Input: part model. Units: mm. Frame: model coordinates. Coordinates: 2 decimals unless noted, no trailing zeros. Write each loop counter-clockwise with the first axis right and the second up, starting at its lowest first coordinate (ties: lowest second). Pieces come first, ordered by that corner, then holes.
1) Section query B-B (y = 10). Output: boundary loops of the cut face in (x, z), then the cut area to 3 significant figures.
2) Line query: L1, parallel to Y at x = 65.75, z = 4.25; L2, parallel to Y at x = 127, z = 4.25; L3, parallel to Y at x = 102.5, z = 1. Output: solid intervals per line, ascending.
3) Pin query (flat end, axial travel): pin 1 Ø2.5 at (x, y) = (-5.06, 36) entering from -Z; pin 2 Ø0.6 at (x, z) = (150.5, 1.5) entering from -Y; pin 3 Ø2 at (x, y) = (45, 14.5) entering from +Z; pin 4 Ø1 at (y, z) = (-24.5, 1.5) entering from -X. Return the tip coordinate at first contact, or that it passes through.
4) Section query C-C (z = 4.25). State how many separate pieces and enclosed holes the cut face has, then the cut area to 3 significant figures.
5) Section query A-A (x = 123). Output: boundary loops of the cut face in (y, z), then the cut area to 3 significant figures.
from build123d import *

# Parameters (mm, degrees)
SKETCH_R     = 17.5
PAD_DEPTH    = 2
SKETCH002_W  = 10
SKETCH002_H  = 2
PAD003_DEPTH = 10
SKETCH003_W  = 10
SKETCH003_H  = 2
PAD004_DEPTH = 10
SKETCH006_W  = 10
SKETCH006_H  = 2
PAD007_DEPTH = 10
SKETCH001_R  = 2.5
PAD006_DEPTH = 5
SKETCH005_R  = 1.5
POCKET_DEPTH = 7.001


with BuildPart() as part:
    # Sketch → Pad (new body)
    with BuildSketch(Plane.XY):
        Polygon((0, 0), (0, 20.5), (0, 41), (20.5, 41), (41, 41), (61.5, 41), (82, 41), (102.5, 41), (82, 41), (102.5, 41), (123, 41), (143.5, 41), (164, 41), (164, 20.5), (164, 0), (143.5, 0), (143.5, -20.5), (143.5, -41), (123, -41), (102.5, -41), (82, -41), (61.5, -41), (41, -41), (20.5, -41), (20.5, -20.5), (20.5, 0), align=None)
        with Locations((20.5, 20.5)):
            Circle(SKETCH_R, mode=Mode.SUBTRACT)
        with Locations((61.5, 20.5)):
            Circle(SKETCH_R, mode=Mode.SUBTRACT)
        with Locations((102.5, 20.5)):
            Circle(SKETCH_R, mode=Mode.SUBTRACT)
        with Locations((143.5, 20.5)):
            Circle(SKETCH_R, mode=Mode.SUBTRACT)
        with Locations((41, -20.5)):
            Circle(SKETCH_R, mode=Mode.SUBTRACT)
        with Locations((82, -20.5)):
            Circle(SKETCH_R, mode=Mode.SUBTRACT)
        with Locations((123, -20.5)):
            Circle(SKETCH_R, mode=Mode.SUBTRACT)
    extrude(amount=PAD_DEPTH)

    # Sketch002 → Pad003 (join)
    with BuildSketch(Plane(origin=(0, 0, 0), x_dir=(0, -1, 0), z_dir=(-1, 0, 0))):
        with Locations((-36, 1)):
            Rectangle(SKETCH002_W, SKETCH002_H)
    extrude(amount=PAD003_DEPTH)

    # Sketch003 (on Face14 of Pad003) → Pad004 (join)
    with BuildSketch(Plane.XZ.offset(41)):
        with Locations((138.5, 1)):
            Rectangle(SKETCH003_W, SKETCH003_H)
    extrude(amount=PAD004_DEPTH)

    # Sketch006 (on Face8 of Pad004) → Pad007 (join)
    with BuildSketch(Plane(origin=(0, 41, 0), x_dir=(-1, 0, 0), z_dir=(0, 1, 0))):
        with Locations((-159, 1)):
            Rectangle(SKETCH006_W, SKETCH006_H)
    extrude(amount=PAD007_DEPTH)

    # Sketch001 (on Face35 of Pad) → Pad006 (join)
    with BuildSketch(Plane.XY.offset(2)):
        with Locations((4.25, 36.75)):
            Circle(SKETCH001_R)
        with Locations((36.75, 36.75)):
            Circle(SKETCH001_R)
        with Locations((4.25, 4.25)):
            Circle(SKETCH001_R)
        with Locations((36.75, 4.25)):
            Circle(SKETCH001_R)
        with Locations((45.25, 36.75)):
            Circle(SKETCH001_R)
        with Locations((77.75, 36.75)):
            Circle(SKETCH001_R)
        with Locations((45.25, 4.25)):
            Circle(SKETCH001_R)
        with Locations((77.75, 4.25)):
            Circle(SKETCH001_R)
        with Locations((86.25, 36.75)):
            Circle(SKETCH001_R)
        with Locations((118.75, 36.75)):
            Circle(SKETCH001_R)
        with Locations((86.25, 4.25)):
            Circle(SKETCH001_R)
        with Locations((118.75, 4.25)):
            Circle(SKETCH001_R)
        with Locations((127.25, 36.75)):
            Circle(SKETCH001_R)
        with Locations((159.75, 36.75)):
            Circle(SKETCH001_R)
        with Locations((127.25, 4.25)):
            Circle(SKETCH001_R)
        with Locations((159.75, 4.25)):
            Circle(SKETCH001_R)
        with Locations((24.75, -4.25)):
            Circle(SKETCH001_R)
        with Locations((57.25, -4.25)):
            Circle(SKETCH001_R)
        with Locations((24.75, -36.75)):
            Circle(SKETCH001_R)
        with Locations((57.25, -36.75)):
            Circle(SKETCH001_R)
        with Locations((65.75, -4.25)):
            Circle(SKETCH001_R)
        with Locations((98.25, -4.25)):
            Circle(SKETCH001_R)
        with Locations((65.75, -36.75)):
            Circle(SKETCH001_R)
        with Locations((98.25, -36.75)):
            Circle(SKETCH001_R)
        with Locations((106.75, -4.25)):
            Circle(SKETCH001_R)
        with Locations((139.25, -4.25)):
            Circle(SKETCH001_R)
        with Locations((106.75, -36.75)):
            Circle(SKETCH001_R)
        with Locations((139.25, -36.75)):
            Circle(SKETCH001_R)
    extrude(amount=PAD006_DEPTH)

    # Sketch005 (on Face93 of Pad006) → Pocket (cut, through all)
    with BuildSketch(Plane.XY.offset(7)):
        with Locations((-5.058944, 36)):
            Circle(SKETCH005_R)
        with Locations((4.25, 36.75)):
            Circle(SKETCH005_R)
        with Locations((36.75, 36.75)):
            Circle(SKETCH005_R)
        with Locations((45.25, 36.75)):
            Circle(SKETCH005_R)
        with Locations((77.75, 36.75)):
            Circle(SKETCH005_R)
        with Locations((86.25, 36.75)):
            Circle(SKETCH005_R)
        with Locations((4.25, 4.25)):
            Circle(SKETCH005_R)
        with Locations((36.75, 4.25)):
            Circle(SKETCH005_R)
        with Locations((45.25, 4.25)):
            Circle(SKETCH005_R)
        with Locations((77.75, 4.25)):
            Circle(SKETCH005_R)
        with Locations((86.25, 4.25)):
            Circle(SKETCH005_R)
        with Locations((118.75, 36.75)):
            Circle(SKETCH005_R)
        with Locations((118.75, 4.25)):
            Circle(SKETCH005_R)
        with Locations((127.25, 36.75)):
            Circle(SKETCH005_R)
        with Locations((127.25, 4.25)):
            Circle(SKETCH005_R)
        with Locations((159.75, 36.75)):
            Circle(SKETCH005_R)
        with Locations((159.75, 4.25)):
            Circle(SKETCH005_R)
        with Locations((106.75, -4.25)):
            Circle(SKETCH005_R)
        with Locations((139.25, -4.25)):
            Circle(SKETCH005_R)
        with Locations((139.25, -36.75)):
            Circle(SKETCH005_R)
        with Locations((106.75, -36.75)):
            Circle(SKETCH005_R)
        with Locations((24.75, -4.25)):
            Circle(SKETCH005_R)
        with Locations((57.25, -4.25)):
            Circle(SKETCH005_R)
        with Locations((65.75, -4.25)):
            Circle(SKETCH005_R)
        with Locations((98.25, -4.25)):
            Circle(SKETCH005_R)
        with Locations((24.75, -36.75)):
            Circle(SKETCH005_R)
        with Locations((57.25, -36.75)):
            Circle(SKETCH005_R)
        with Locations((65.75, -36.75)):
            Circle(SKETCH005_R)
        with Locations((98.25, -36.75)):
            Circle(SKETCH005_R)
        with Locations((138.5, -46)):
            Circle(SKETCH005_R)
        with Locations((159, 46)):
            Circle(SKETCH005_R)
    extrude(amount=-POCKET_DEPTH, mode=Mode.SUBTRACT)


solid = part.part
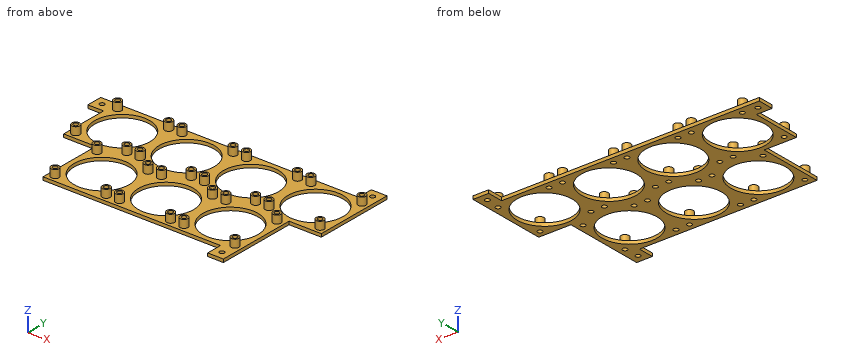
Answer:
1. outline: (0, 0) - (6.5, 0) - (6.5, 2) - (0, 2) - close; (34.5, 0) - (47.5, 0) - (47.5, 2) - (34.5, 2) - close; (75.5, 0) - (88.5, 0) - (88.5, 2) - (75.5, 2) - close; (116.5, 0) - (129.5, 0) - (129.5, 2) - (116.5, 2) - close; (157.5, 0) - (164, 0) - (164, 2) - (157.5, 2) - close
1. area: 104 mm2
2. L1: y = -39.25 to -38.25, -35.25 to -34.25, -6.75 to -5.75, -2.75 to -1.75
2. L2: y = 1.76 to 2.77, 5.73 to 6.74, 34.26 to 35.27, 38.23 to 39.24
2. L3: y = -41 to 3, 38 to 41
3. pin 1: passes through
3. pin 2: stops at y = 0
3. pin 3: stops at z = 2
3. pin 4: stops at x = 20.5
4. separate pieces: 28
4. enclosed holes: 28
4. area: 352 mm2
5. outline: (-41, 0) - (-38, 0) - (-38, 2) - (-41, 2) - close; (-3, 0) - (41, 0) - (41, 2) - (-3, 2) - close
5. area: 94.0 mm2
